```python
from build123d import *

# Parameters (mm, degrees)
SKETCH_R     = 9.5
PAD_DEPTH    = 2
SKETCH001_W  = 2
SKETCH001_H  = 1.5
POCKET_DEPTH = 5
SKETCH002_R  = 10.5
PAD001_DEPTH = 5


with BuildPart() as part:
    # Sketch → Pad (new body)
    with BuildSketch(Plane.XY):
        Circle(SKETCH_R)
    extrude(amount=PAD_DEPTH)

    # Sketch001 (on Face3 of Pad) → Pocket (cut)
    with BuildSketch(Plane.XY.offset(2)):
        with Locations((9.5, 0)):
            Rectangle(SKETCH001_W, SKETCH001_H)
        with Locations((-9.5, 0)):
            Rectangle(SKETCH001_W, SKETCH001_H)
    extrude(amount=-POCKET_DEPTH, mode=Mode.SUBTRACT)

    # Sketch002 (on Face4 of Pocket) → Pad001 (join)
    with BuildSketch(Plane.XY.offset(2)):
        Circle(SKETCH002_R)
    extrude(amount=PAD001_DEPTH)


solid = part.part
```
Source: CAD feature listing. Evaluate the final solid. Frame: model axes, mm. A direction names the side the tool comes from. Round coordinates to 2 decimals unless told otherwise and drop trailing zeros. Loops run counter-clockwise (first coordinate to the right, second up) from the corner with the lowest first, then second, coordinate; pieces in that order, holes last.
(1) Material intervals for probe 1 along X at (y, z) = (0, 1.5); probe 2 along Z at (x, y) = (9, -3.75); probe 3 along Y at (x, z) = (-7, 0.75), sorted ascending.
From the geometry:
probe 1: x = -8.5 to 8.5
probe 2: z = 2 to 7
probe 3: y = -6.42 to 6.42
(2) Access query for faces 1 (the flat face through (0, 0, 7)), 2 (the flat face through (-9, 0.75, 1)), 3 (the flat face through (9, -0.75, 1)). Directions: +Z, -Z, +X, -X, +Y, -Y. A direction counts if a zero-diameter tool reaches every point of the face in a straight line with its end or side. Return the directions, or none.
From the geometry:
face 1: +Z, +X, -X, +Y, -Y
face 2: -Z, -X
face 3: -Z, +X
(3) Section query B-B (x = 0). Output: boundary loops of the cut face in (y, z), and give its area (3 significant figures).
From the geometry:
outline: (-10.5, 2) - (-9.5, 2) - (-9.5, 0) - (9.5, 0) - (9.5, 2) - (10.5, 2) - (10.5, 7) - (-10.5, 7) - close
area: 143 mm2
(4) Contact query for flat-ended pins moving along their axis: pin 1 Ø1.2 at (y, z) = (-0.5, 1) entering from +X; pin 2 Ø0.8 at (y, z) = (-0.5, 1) entering from -X; pin 3 Ø0.8 at (x, z) = (-9, 1) entering from +Y. Output: stop coordinate, or through.
From the geometry:
pin 1: stops at x = 9.47
pin 2: stops at x = -9.47
pin 3: stops at y = 4.04
(5) Section query A-A (y = 0). Output: boundary loops of the cut face in (x, z), and give its area (3 significant figures).
From the geometry:
outline: (-10.5, 2) - (-8.5, 2) - (-8.5, 0) - (8.5, 0) - (8.5, 2) - (10.5, 2) - (10.5, 7) - (-10.5, 7) - close
area: 139 mm2
(6) Section query C-C (z = 6.5). Output: boundary loops of the cut face in (x, y).
From the geometry:
outline: circle Ø21 at (0, 0)
(7) Pull-direction query (Y, two-part tool) for faces 4 (the cylindrical face through (0.198, 9.498, 0.986)), 5 (the flat face through (0, 0, 0)), 6 (the cylindrical face through (-0.198, -9.498, 0.986)), 7 (the flat face through (8.5, 0, 1)); classes: +Y half, -Y half, draft (parallel to the pull), parting line (faces both ways), or undercut.
From the geometry:
face 4: +Y half
face 5: draft
face 6: -Y half
face 7: undercut
